Here's how the part is built. I have some questions about the finished solid (model axes, mm). Coordinates: 2 decimals unless noted, no trailing zeros. Loops run counter-clockwise (first coordinate to the right, second up) from the corner with the lowest first, then second, coordinate; pieces in that order, holes last. Notation, with made-up numbers: (-32.75, 19.25) -> (-26.75, 19.25) arc R17 cw to (-26.75, 36.25) -> close; hole circle Ø8 at (68.25, 78.25). An arc over 180 degrees is marked (long way). Answer as a JSON object with one key per item and string values. Group by question number.
Q1. I'm going to push flat-ended pins straight in: pin 1 (6 mm diameter, centred on x = -35.5, z = 37, fed in from +Y); pin 2 (0.8 mm diameter, centred on y = 0.5, z = -30, fed in from -X); pin 3 (0.8 mm diameter, centred on y = 0.5, z = -22.5, fed in from +X). Where does each tip first touch, or does it pass through?
Q2. I need wall thicknesses on line 1 (Z direction, x = -9.5, y = 0.9); line 2 (Z direction, x = 0, y = 0.7) (3 decimals); line 3 (X direction, y = 0.6, z = -30.5) (1 decimal). Which ranges of each line are inside material? Lowest first, please.
Q3. I want a section at A-A on x = 0. Write out the boundary of the cut face in (y, z) (3 decimals), then the cut area to 3 significant figures.
Q4. I want a section at D-D on x = -21.5. Write out the boundary of the cut face in (y, z), then the cut area to 3 significant figures.
Q5. I want a section at B-B on x = 32. Write out the boundary of the cut face in (y, z).
Q6. I want a section at C-C on y = 1.15. Count the separate pieces of the cut face and the enclosed holes in it, then the cut area to 3 significant figures.
Q7. Thinking about a two-plate mould opening in Z: for faces 1 (the cylindrical face through (-37.794, 0.751, 28.979)), 2 (the cylindrical face through (2.623, 0.751, 43.345)), 3 (the flat face through (0, 1.524, 7)), which applies, released by +Z, released by -Z, zero draft, split by the parting line, or undercut?
```python
from build123d import *

# Parameters (mm, degrees)
SKETCH1_R           = 47.625
SKETCH1_R_2         = 5.08
BOSS_EXTRUDE1_DEPTH = 1.524


with BuildPart() as part:
    # Sketch1 → Boss-Extrude1 (new body)
    with BuildSketch(Plane(origin=(0, 0, 0), x_dir=(1, 0, 0), z_dir=(0, 1, 0))):
        Circle(SKETCH1_R)
        Circle(SKETCH1_R_2, mode=Mode.SUBTRACT)
        with BuildLine():
            Line((1.5875, 40.999319735), (1.5875, 10.390548289))
            ThreePointArc((1.5875, 10.390548289), (2.090339318, 8.675852313), (3.439583333, 7.504284876))
            ThreePointArc((3.439583333, 7.504284876), (4.1275, 7.149039708), (4.779109673, 6.730908983))
            ThreePointArc((4.779109673, 6.730908983), (6.468338843, 6.148213109), (8.204728778, 6.570089473))
            Line((8.204728778, 6.570089473), (34.712702429, 21.874475196))
            ThreePointArc((34.712702429, 21.874475196), (36.234379788, 23.980956457), (35.673294923, 26.518267842))
            ThreePointArc((35.673294923, 26.518267842), (22.225, 38.494829198), (5.128846154, 44.153113561))
            ThreePointArc((5.128846154, 44.153113561), (2.650927605, 43.370371616), (1.5875, 40.999319735))
        make_face(mode=Mode.SUBTRACT)
        with BuildLine():
            Line((36.300202429, 19.124844539), (9.792228778, 3.820458816))
            ThreePointArc((9.792228778, 3.820458816), (8.558678162, 2.527639204), (8.218693006, 0.773375893))
            ThreePointArc((8.218693006, 0.773375893), (8.255, 0), (8.218693006, -0.773375893))
            ThreePointArc((8.218693006, -0.773375893), (8.558678162, -2.527639204), (9.792228778, -3.820458816))
            Line((9.792228778, -3.820458816), (36.300202429, -19.124844539))
            ThreePointArc((36.300202429, -19.124844539), (38.885307393, -19.389415159), (40.802141077, -17.634845719))
            ThreePointArc((40.802141077, -17.634845719), (44.45, 0), (40.802141077, 17.634845719))
            ThreePointArc((40.802141077, 17.634845719), (38.885307393, 19.389415159), (36.300202429, 19.124844539))
        make_face(mode=Mode.SUBTRACT)
        with BuildLine():
            Line((34.712702429, -21.874475196), (8.204728778, -6.570089473))
            ThreePointArc((8.204728778, -6.570089473), (6.468338843, -6.148213109), (4.779109673, -6.730908983))
            ThreePointArc((4.779109673, -6.730908983), (4.1275, -7.149039708), (3.439583333, -7.504284876))
            ThreePointArc((3.439583333, -7.504284876), (2.090339318, -8.675852313), (1.5875, -10.390548289))
            Line((1.5875, -10.390548289), (1.5875, -40.999319735))
            ThreePointArc((1.5875, -40.999319735), (2.650927605, -43.370371616), (5.128846154, -44.153113561))
            ThreePointArc((5.128846154, -44.153113561), (22.225, -38.494829198), (35.673294923, -26.518267842))
            ThreePointArc((35.673294923, -26.518267842), (36.234379788, -23.980956457), (34.712702429, -21.874475196))
        make_face(mode=Mode.SUBTRACT)
        with BuildLine():
            Line((-1.5875, -40.999319735), (-1.5875, -10.390548289))
            ThreePointArc((-1.5875, -10.390548289), (-2.090339318, -8.675852313), (-3.439583333, -7.504284876))
            ThreePointArc((-3.439583333, -7.504284876), (-4.1275, -7.149039708), (-4.779109673, -6.730908983))
            ThreePointArc((-4.779109673, -6.730908983), (-6.468338843, -6.148213109), (-8.204728778, -6.570089473))
            Line((-8.204728778, -6.570089473), (-34.712702429, -21.874475196))
            ThreePointArc((-34.712702429, -21.874475196), (-36.234379788, -23.980956457), (-35.673294923, -26.518267842))
            ThreePointArc((-35.673294923, -26.518267842), (-22.225, -38.494829198), (-5.128846154, -44.153113561))
            ThreePointArc((-5.128846154, -44.153113561), (-2.650927605, -43.370371616), (-1.5875, -40.999319735))
        make_face(mode=Mode.SUBTRACT)
        with BuildLine():
            Line((-36.300202429, -19.124844539), (-9.792228778, -3.820458816))
            ThreePointArc((-9.792228778, -3.820458816), (-8.558678162, -2.527639204), (-8.218693006, -0.773375893))
            ThreePointArc((-8.218693006, -0.773375893), (-8.255, 0), (-8.218693006, 0.773375893))
            ThreePointArc((-8.218693006, 0.773375893), (-8.558678162, 2.527639204), (-9.792228778, 3.820458816))
            Line((-9.792228778, 3.820458816), (-36.300202429, 19.124844539))
            ThreePointArc((-36.300202429, 19.124844539), (-38.885307393, 19.389415159), (-40.802141077, 17.634845719))
            ThreePointArc((-40.802141077, 17.634845719), (-44.45, 0), (-40.802141077, -17.634845719))
            ThreePointArc((-40.802141077, -17.634845719), (-38.885307393, -19.389415159), (-36.300202429, -19.124844539))
        make_face(mode=Mode.SUBTRACT)
        with BuildLine():
            Line((-34.712702429, 21.874475196), (-8.204728778, 6.570089473))
            ThreePointArc((-8.204728778, 6.570089473), (-6.468338843, 6.148213109), (-4.779109673, 6.730908983))
            ThreePointArc((-4.779109673, 6.730908983), (-4.1275, 7.149039708), (-3.439583333, 7.504284876))
            ThreePointArc((-3.439583333, 7.504284876), (-2.090339318, 8.675852313), (-1.5875, 10.390548289))
            Line((-1.5875, 10.390548289), (-1.5875, 40.999319735))
            ThreePointArc((-1.5875, 40.999319735), (-2.650927605, 43.370371616), (-5.128846154, 44.153113561))
            ThreePointArc((-5.128846154, 44.153113561), (-22.225, 38.494829198), (-35.673294923, 26.518267842))
            ThreePointArc((-35.673294923, 26.518267842), (-36.234379788, 23.980956457), (-34.712702429, 21.874475196))
        make_face(mode=Mode.SUBTRACT)
    extrude(amount=BOSS_EXTRUDE1_DEPTH)


solid = part.part
```
Result set:
{
 "1": {"pin 1": "passes through", "pin 2": "stops at x = -37.31", "pin 3": "stops at x = 42.19"},
 "2": {"line 1": "z = -46.67 to -43.42, -7.32 to -3.63, 3.63 to 7.32, 43.42 to 46.67", "line 2": "z = -47.625 to -5.08, 5.08 to 47.625", "line 3": "x = -36.6 to -32.3, -1.6 to 1.6, 32.3 to 36.6"},
 "3": {"outline": "(0, -47.625) -> (1.524, -47.625) -> (1.524, -5.08) -> (0, -5.08) -> close; (0, 5.08) -> (1.524, 5.08) -> (1.524, 47.625) -> (0, 47.625) -> close", "area": "130 mm²"},
 "4": {"outline": "(0, -42.5) -> (1.52, -42.5) -> (1.52, -38.9) -> (0, -38.9) -> close; (0, -14.25) -> (1.52, -14.25) -> (1.52, -10.58) -> (0, -10.58) -> close; (0, 10.58) -> (1.52, 10.58) -> (1.52, 14.25) -> (0, 14.25) -> close; (0, 38.9) -> (1.52, 38.9) -> (1.52, 42.5) -> (0, 42.5) -> close", "area": "22.1 mm²"},
 "5": {"outline": "(0, -35.27) -> (1.52, -35.27) -> (1.52, -30.85) -> (0, -30.85) -> close; (0, -20.31) -> (1.52, -20.31) -> (1.52, -16.64) -> (0, -16.64) -> close; (0, 16.64) -> (1.52, 16.64) -> (1.52, 20.31) -> (0, 20.31) -> close; (0, 30.85) -> (1.52, 30.85) -> (1.52, 35.27) -> (0, 35.27) -> close"},
 "6": {"separate pieces": "1", "enclosed holes": "7", "area": "1,780 mm²"},
 "7": {"face 1": "split by the parting line", "face 2": "undercut", "face 3": "zero draft"}
}
